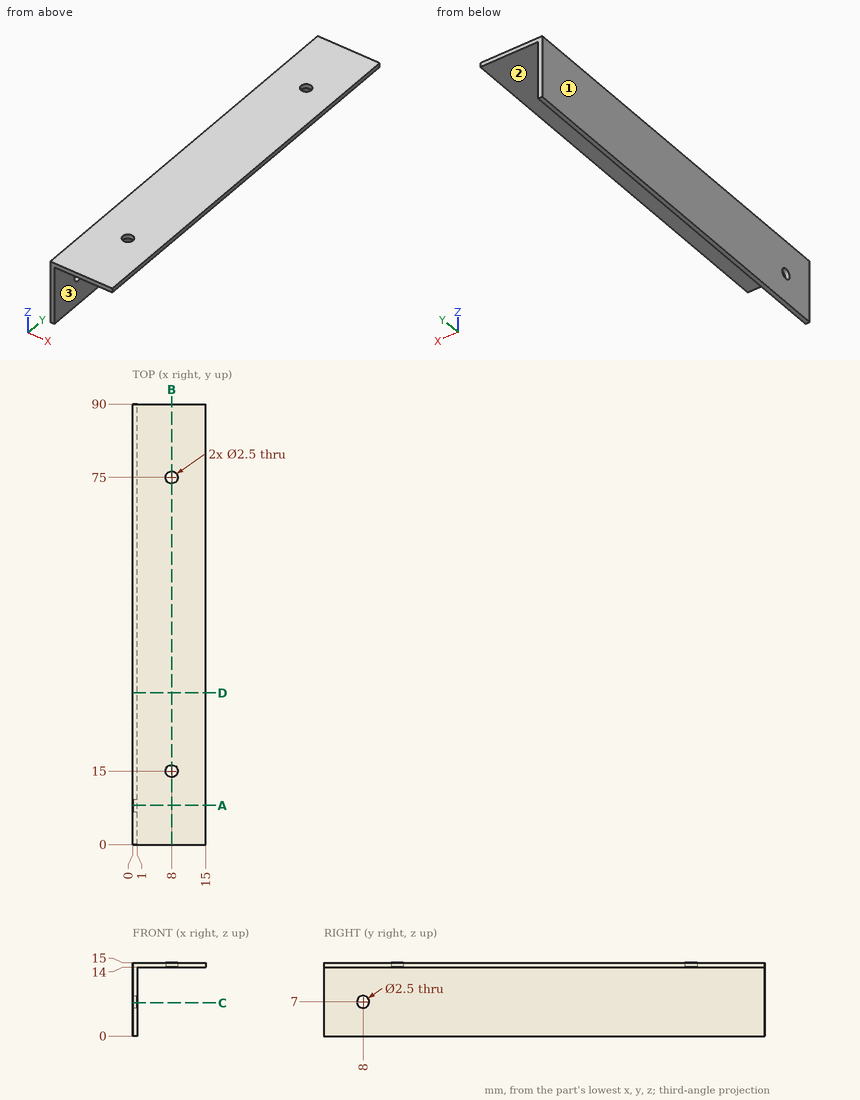
Can you work these out from the drawing? Everything is in mm from the part's minimum corner. Round coordinates to 2 decimals unless told otherwise and drop trailing zeros. Write each loop counter-clockwise with the first axis right and the second up, starting at its lowest first coordinate (ties: lowest second). Pieces come first, ordered by that corner, then holes.
1. Suppose I cut it at A-A (y = 8). List the corners of the cut face in (x, z) for me, and give its area (3 significant figures).
2. Suppose I cut it at B-B (x = 8). List the corners of the cut face in (y, z) for me.
3. I need wall thicknesses on L1, parallel to Y at x = 8, z = 14.2; L2, parallel to Y at x = 0.5, z = 7; L3, parallel to X at y = 75, z = 5.5. Which ranges of each line are inside material? Lowest first, please.
4. Will these pins go through, and if not, where does the flat tip stop? pin 1 Ø4 at (y, z) = (8, 7) entering from +X; pin 2 Ø3 at (x, y) = (8, 15) entering from -Z; pin 3 Ø2 at (x, y) = (8, 75) entering from -Z.
5. Suppose I cut it at C-C (z = 6.75). List the corners of the cut face in (x, y) for me, and give its area (3 significant figures).
6. If we mould it in two halves opening along X, with no side actions, what happens to the marked faces 1, 2 and 3? For each: released by +X, released by -X, zero draft, split by the parting line, or undercut.
7. Suppose I cut it at D-D (y = 31). List the corners of the cut face in (x, z) for me.
Answer sheet:
1. outline: (0, 0) - (1, 0) - (1, 5.75) - (0, 5.75) - close; (0, 8.25) - (1, 8.25) - (1, 14) - (15, 14) - (15, 15) - (0, 15) - close
1. area: 26.5 mm2
2. outline: (0, 14) - (13.75, 14) - (13.75, 15) - (0, 15) - close; (16.25, 14) - (73.75, 14) - (73.75, 15) - (16.25, 15) - close; (76.25, 14) - (90, 14) - (90, 15) - (76.25, 15) - close
3. L1: y = 0 to 13.75, 16.25 to 73.75, 76.25 to 90
3. L2: y = 0 to 6.75, 9.25 to 90
3. L3: x = 0 to 1
4. pin 1: stops at x = 1
4. pin 2: stops at z = 14
4. pin 3: passes through
5. outline: (0, 0) - (1, 0) - (1, 6.78) - (0, 6.78) - close; (0, 9.22) - (1, 9.22) - (1, 90) - (0, 90) - close
5. area: 87.6 mm2
6. face 1: released by -X
6. face 2: zero draft
6. face 3: released by +X
7. outline: (0, 0) - (1, 0) - (1, 14) - (15, 14) - (15, 15) - (0, 15) - close
